Job drawing, mm, ordinate dimensions from the low corner. One solid piece. Round coordinates to 2 decimals unless told otherwise and drop trailing zeros. Loops run counter-clockwise (first coordinate to the right, second up) from the corner with the lowest first, then second, coordinate; pieces in that order, holes last.
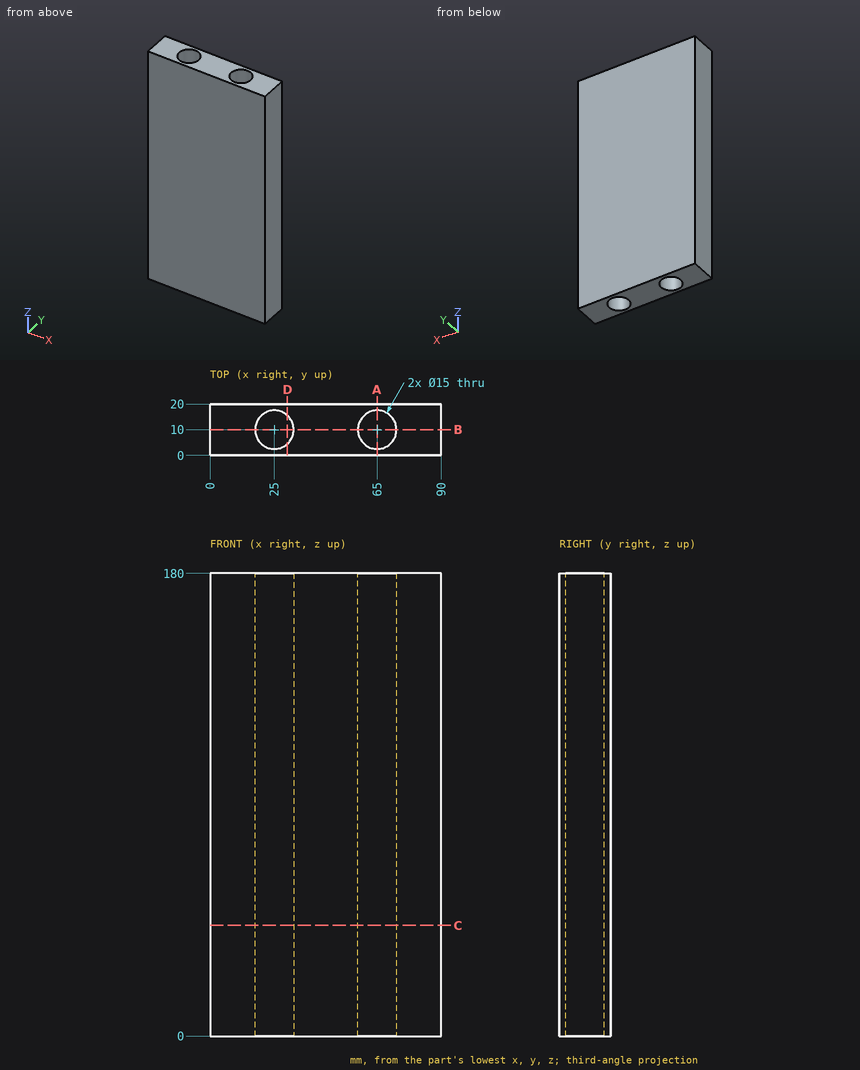
Item 1: Cut at C-C, the plane z = 43. Give the cut face in (x, y), plus the area to 3 significant figures.
Answers follow:
outline: (0, 0) - (90, 0) - (90, 20) - (0, 20) - close; hole circle Ø15 at (25, 10); hole circle Ø15 at (65, 10)
area: 1,450 mm2
Item 2: Flat gauge pins, fed straight in: P1, Ø1.5, axis at y = 4.5, z = 144.5, coming from the -X side; P2, Ø9, axis at x = 25, y = 10, coming from the +Z side. Where does each tip first touch, or does it go through?
Answers follow:
P1: stops at x = 0
P2: passes through
Item 3: Cut at B-B, the plane y = 10. Give the cut face in (x, z).
Answers follow:
outline: (0, 0) - (17.5, 0) - (17.5, 180) - (0, 180) - close; (32.5, 0) - (57.5, 0) - (57.5, 180) - (32.5, 180) - close; (72.5, 0) - (90, 0) - (90, 180) - (72.5, 180) - close
Item 4: Cut at D-D, the plane x = 30. Give the cut face in (y, z), plus the area to 3 significant figures.
Answers follow:
outline: (0, 0) - (4.41, 0) - (4.41, 180) - (0, 180) - close; (15.59, 0) - (20, 0) - (20, 180) - (15.59, 180) - close
area: 1,590 mm2
Item 5: Probe line 1 (Y direction, x = 25, z = 101.5); line 2 (X direction, y = 13.5, z = 168); line 3 (X direction, y = 7.75, z = 167). List the from-to ranges inside material, lowest first.
Answers follow:
line 1: y = 0 to 2.5, 17.5 to 20
line 2: x = 0 to 18.37, 31.63 to 58.37, 71.63 to 90
line 3: x = 0 to 17.85, 32.15 to 57.85, 72.15 to 90
Item 6: Cut at A-A, the plane x = 65. Give the cut face in (y, z), plus the area to 3 significant figures.
Answers follow:
outline: (0, 0) - (2.5, 0) - (2.5, 180) - (0, 180) - close; (17.5, 0) - (20, 0) - (20, 180) - (17.5, 180) - close
area: 900 mm2
